```python
from build123d import *

# Parameters (mm, degrees)
SKETCH1_R           = 2.9083
SKETCH1_R_2         = 1.524
BOSS_EXTRUDE1_DEPTH = 32.131
BOSS_EXTRUDE5_START = -0.635
SKETCH7_R           = 1.524
SKETCH7_R_2         = 1.190625
BOSS_EXTRUDE5_DEPTH = 0.635
SKETCH8_R           = 1.7859375
CUT_EXTRUDE2_DEPTH  = 3.175


with BuildPart() as part:
    # Sketch1 → Boss-Extrude1 (new body)
    with BuildSketch(Plane(origin=(0, 0, 0), x_dir=(1, 0, 0), z_dir=(0, 1, 0))):
        with Locations(Location((0, 0, 0), (0, 0, 270))):
            Circle(SKETCH1_R)
        with Locations(Location((0, 0, 0), (0, 0, 270))):
            Circle(SKETCH1_R_2, mode=Mode.SUBTRACT)
    extrude(amount=BOSS_EXTRUDE1_DEPTH)

    # Sketch7 → Boss-Extrude5 (add)
    with BuildSketch(Plane(origin=(0, 32.131, 0), x_dir=(1, 0, 0), z_dir=(0, 1, 0)).offset(BOSS_EXTRUDE5_START)):
        with Locations(Location((0, 0, 0), (0, 0, 270))):
            Circle(SKETCH7_R)
        with Locations(Location((0, 0, 0), (0, 0, 270))):
            Circle(SKETCH7_R_2, mode=Mode.SUBTRACT)
    extrude(amount=BOSS_EXTRUDE5_DEPTH)

    # Sketch8 → Cut-Extrude2 (cut)
    with BuildSketch(Plane(origin=(0, 31.496, 0), x_dir=(1, 0, 0), z_dir=(0, 1, 0))):
        with Locations(Location((0, 0, 0), (0, 0, 270))):
            Circle(SKETCH8_R)
    extrude(amount=-CUT_EXTRUDE2_DEPTH, mode=Mode.SUBTRACT)


solid = part.part
```
Build history of the part. All positions in model axes, mm. A direction names the side the tool comes from. Round coordinates to 2 decimals unless told otherwise and drop trailing zeros. Order: outer loops, then holes, each group sorted by start corner. A loop starts at its lowest first (then second) coordinate and runs counter-clockwise, first axis right, second up. Notation, with made-up numbers: (59.25, -32) - (74.25, -32) arc R11 cw to (74.25, -18) - close; hole circle Ø3 at (86, -0.75). An arc over 180 degrees is marked (long way). Use a Markdown table: item, result.
1) Saw through at C-C on y = 18. Write the cut outline in (x, z).
Recorded:
| item | result |
|---|---|
| outline | circle Ø5.82 at (0, 0); hole circle Ø3.05 at (0, 0) |
2) Wall check: L1, parallel to X at y = 19.5, z = 0; L2, parallel to X at y = 29.4, z = 0; L3, parallel to Z at x = 0.15, y = 14.5. Give the ranges that are in metal, low to high.
Recorded:
| item | result |
|---|---|
| L1 | x = -2.91 to -1.52, 1.52 to 2.91 |
| L2 | x = -2.91 to -1.79, 1.79 to 2.91 |
| L3 | z = -2.9 to -1.52, 1.52 to 2.9 |
3) Tool access for faces 4 (the face through (1.285, 13.962, 0.819)), 5 (the face through (-0.724, 31.809, -0.945)): list every direction of +Z, -Z, +X, -X, +Y, -Y with a clear straight run to the whole face (end or side of a thin tool).
Recorded:
| item | result |
|---|---|
| face 4 | -Y |
| face 5 | +Y, -Y |
4) Saw through at B-B on x = 0. Write the cut outline in (y, z).
Recorded:
| item | result |
|---|---|
| outline | (0, -2.91) - (32.13, -2.91) - (32.13, -1.19) - (31.5, -1.19) - (31.5, -1.79) - (28.32, -1.79) - (28.32, -1.52) - (0, -1.52) - close; (0, 1.52) - (28.32, 1.52) - (28.32, 1.79) - (31.5, 1.79) - (31.5, 1.19) - (32.13, 1.19) - (32.13, 2.91) - (0, 2.91) - close |
5) Pull direction X, two halves, no side cores. Call faces 1 (the face through (0.079, 29.931, -1.784)), 2 (the face through (0.874, 15.841, 2.774)), 3 (the face through (-1, 32.131, 1)): pulls with the +X half, pulls with the -X half, needs draft (parallel to the pull), parting line crosses it, or undercut.
Recorded:
| item | result |
|---|---|
| face 1 | undercut |
| face 2 | parting line crosses it |
| face 3 | needs draft |
6) Saw through at D-D on z = 2.1. Write the cut outline in (x, y).
Recorded:
| item | result |
|---|---|
| outline | (-2.01, 0) - (2.01, 0) - (2.01, 32.13) - (-2.01, 32.13) - close |
7) Flat gauge pins, fed straight in: pin 1 Ø1.5 at (y, z) = (9.5, 1) entering from -X; pin 2 Ø1.1 at (x, z) = (0.5, 0.5) entering from -Y. Where does each tip first touch, or does it go through?
Recorded:
| item | result |
|---|---|
| pin 1 | stops at x = -2.9 |
| pin 2 | stops at y = 31.5 |
8) Saw through at A-A on z = 0. Write the cut outline in (x, y), and give its area (3 significant figures).
Recorded:
| item | result |
|---|---|
| outline | (-2.91, 0) - (-1.52, 0) - (-1.52, 28.32) - (-1.79, 28.32) - (-1.79, 31.5) - (-1.19, 31.5) - (-1.19, 32.13) - (-2.91, 32.13) - close; (1.19, 31.5) - (1.79, 31.5) - (1.79, 28.32) - (1.52, 28.32) - (1.52, 0) - (2.91, 0) - (2.91, 32.13) - (1.19, 32.13) - close |
| area | 87.7 mm² |
